CAD build for the part. Positions are in the model's coordinates, mm. A direction names the side the tool comes from. Round coordinates to 2 decimals unless told otherwise and drop trailing zeros. Use one line per item in the form item = value.
from build123d import *

# Parameters (mm, degrees)
F0_W     = 200
F0_H     = 800
F1_DEPTH = 40
F3_DEPTH = 4


# Not quite as in the source:
# - ends of sketch curves that miss each other by under 0.0002 mm in the source are joined
# - a feature of the source that left no trace in its solid (it failed there, or was rolled back) is left out


with BuildPart() as f1:
    # F0 (on Top) → F1 (new body)
    with BuildSketch(Plane.XY):
        with Locations((100, 400)):
            Rectangle(F0_W, F0_H)
    extrude(amount=-F1_DEPTH)

    # F2 (on face) → F3 (cut)
    with BuildSketch(Plane.XY):
        with BuildLine():
            add(Edge.make_bspline(
                [(74.0144076195, 49.4648806587), (79.2780666431, 43.995087588), (85.5330334882, 36.6035044423), (93.9858326346, 24.9514187131)],
                knots=[0, 0, 0, 0, 1, 1, 1, 1], degree=3))
            Line((93.9858326346, 24.9514187131), (124.8743034899, 24.9514187131))
            add(Edge.make_bspline(
                [(124.8743034899, 24.9514187131), (117.373795502, 30.8557542171), (100.1070204646, 40.4994924549), (85.0477587545, 51.6157174292)],
                knots=[0, 0, 0, 0, 1, 1, 1, 1], degree=3))
            add(Edge.make_bspline(
                [(85.0477587545, 51.6157174292), (78.3221982923, 56.5802620007), (72.0369383461, 61.8389475301), (67.2585806524, 67.1891107778)],
                knots=[0, 0, 0, 0, 1, 1, 1, 1], degree=3))
            add(Edge.make_bspline(
                [(67.2585806524, 67.1891107778), (64.0111017086, 70.825439839), (61.4596060965, 74.5036446576), (59.9390200859, 78.1614235749)],
                knots=[0, 0, 0, 0, 1, 1, 1, 1], degree=3))
            add(Edge.make_bspline(
                [(59.9390200859, 78.1614235749), (58.6848351698, 81.1781536647), (58.1318996379, 84.1804553021), (58.4680892286, 87.1331416805)],
                knots=[0, 0, 0, 0, 1, 1, 1, 1], degree=3))
            add(Edge.make_bspline(
                [(58.4680892286, 87.1331416805), (58.8494259124, 90.279355495), (60.7095393399, 92.4826134262), (63.6064002406, 92.9386057154)],
                knots=[0, 0, 0, 0, 1, 1, 1, 1], degree=3))
            add(Edge.make_bspline(
                [(63.6064002406, 92.9386057154), (66.1469914002, 93.338307093), (69.4850038962, 92.3950054588), (73.3222940387, 89.5654596054)],
                knots=[0, 0, 0, 0, 1, 1, 1, 1], degree=3))
            Line((73.3222940387, 89.5654596054), (73.3850611313, 116.1375625051))
            add(Edge.make_bspline(
                [(73.3850611313, 116.1375625051), (61.2635786151, 114.5669223978), (16.5941537425, 105.3232312885), (51.4149430547, 70.5446634846)],
                knots=[0, 0, 0, 0, 1, 1, 1, 1], degree=3))
            add(Edge.make_bspline(
                [(51.4149430547, 70.5446634846), (59.7059440621, 62.0496960224), (65.5907579364, 58.2180974722), (74.0144076195, 49.4648806587)],
                knots=[0, 0, 0, 0, 1, 1, 1, 1], degree=3))
        make_face()
        with BuildLine():
            add(Edge.make_bspline(
                [(91.6621868878, 90.8201365516), (86.9476734338, 98.0875153234), (81.3030633718, 105.4382865607), (76.6022868683, 111.646603626)],
                knots=[0, 0, 0, 0, 1, 1, 1, 1], degree=3))
            Line((76.6022868683, 111.646603626), (76.7011849335, 87.2598062052))
            add(Edge.make_bspline(
                [(76.7011849335, 87.2598062052), (83.8706497004, 81.3502046486), (97.2544954721, 67.4086626207), (84.6318469774, 55.4167037236)],
                knots=[0, 0, 0, 0, 1, 1, 1, 1], degree=3))
            add(Edge.make_bspline(
                [(84.6318469774, 55.4167037236), (87.753206619, 52.954491641), (90.1454573299, 51.1927975466), (93.6734466659, 48.8385927365)],
                knots=[0, 0, 0, 0, 1, 1, 1, 1], degree=3))
            add(Edge.make_bspline(
                [(93.6734466659, 48.8385927365), (99.7215214715, 54.7664924964), (102.6407232018, 62.4339183966), (101.2052451133, 70.0858652935)],
                knots=[0, 0, 0, 0, 1, 1, 1, 1], degree=3))
            add(Edge.make_bspline(
                [(101.2052451133, 70.0858652935), (100.3360804582, 76.0348691585), (96.4859975312, 83.3838717469), (91.6621868878, 90.8201365516)],
                knots=[0, 0, 0, 0, 1, 1, 1, 1], degree=3))
        make_face()
        with BuildLine():
            add(Edge.make_bspline(
                [(71.9907407021, 47.2640828783), (51.4723643059, 39.233897758), (44.7548226057, 48.169378506), (42.5680809306, 50.3631415847)],
                knots=[0, 0, 0, 0, 1, 1, 1, 1], degree=3))
            Line((42.5680809306, 50.3631415847), (24.8743034899, 28.961757198))
            add(Edge.make_bspline(
                [(24.8743034899, 28.961757198), (35.1755403208, 28.6025219778), (57.6930087218, 28.8069538664), (79.2330525311, 38.8320952786)],
                knots=[0, 0, 0, 0, 1, 1, 1, 1], degree=3))
            add(Edge.make_bspline(
                [(79.2330525311, 38.8320952786), (77.1638794716, 41.6785297354), (74.3423390821, 44.7962323959), (71.9907407021, 47.2640828783)],
                knots=[0, 0, 0, 0, 1, 1, 1, 1], degree=3))
        make_face()
    extrude(amount=-F3_DEPTH, mode=Mode.SUBTRACT)


solid = f1.part
1) Drill centre line: probe 1 along Y at (x, z) = (122.5, -2). Where is it in solid material? Low to high.
Report:
probe_1 = 0 to 24.95, 26.72 to 800
2) Flat gauge pin, fed straight in: pin 1 (10.5 mm diameter, centred on x = 48, y = 37, fed in from +Z). Where does the tip first touch, or does it go through?
Report:
pin_1 = -4
3) Tool access for faces 1 (the flat face through (99, 406, 0)), 2 (the flat face through (52, 37, -4)): list every direction of +Z, -Z, +X, -X, +Y, -Y with a clear straight run to the whole face (end or side of a thin tool).
Report:
face_1 = +Z, +X, -X, +Y, -Y
face_2 = +Z
4) Two-plate mould, pull along X, no slides. Class faces 3 (the flat face through (99, 800, -20)), 4 (the flat face through (89, 81, -4)), 5 (the flat face through (200, 394, -20)): +X half, -X half, draft (parallel to the pull), parting line (faces both ways), or undercut.
Report:
face_3 = draft
face_4 = undercut
face_5 = +X half
